The figure shows three views and two pictorial views of one solid part (mm, origin at its lowest corner). Answer the questions. Give positions to 0.01 mm unless a question says otherwise; leave off trailing zeros. Order: outer loops, then holes, each group sorted by start corner. A loop starts at its lowest first (then second) coordinate and runs counter-clockwise, first axis right, second up. Notation, with made-up numbers: (-19, -35) - (5, -35) arc R29 cw to (5, -15) - close; hole circle Ø5 at (1, 28). An arc over 180 degrees is marked (long way). Return JSON: item names as keys, results as strings. Group by question number.
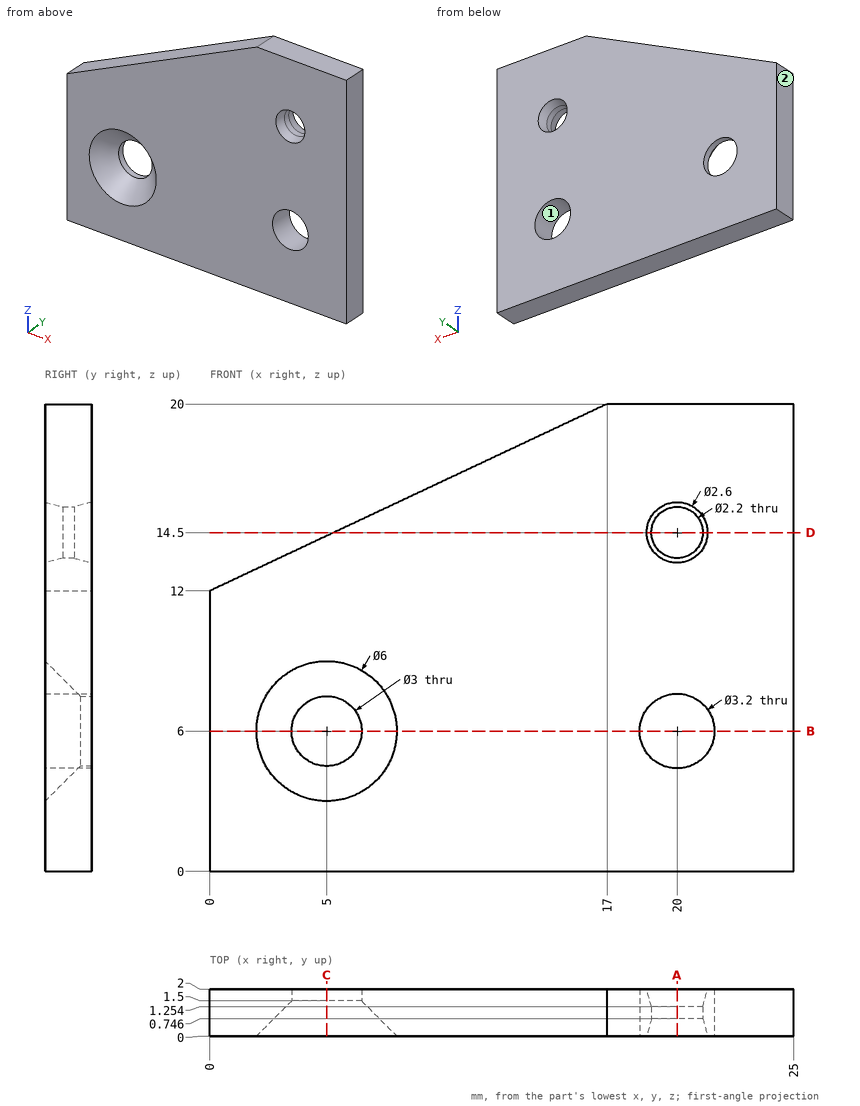
1. This flat-tipped pin is pushed along its axis until it touches: pin 1 (3 mm diameter, centred on x = 20, z = 14.5, fed in from +Y). Where does it stop, or does it pass through?
2. The part is cut by section D-D (z = 14.5). Give the vertices of the cut face in (x, y).
3. The part is cut by section A-A (x = 20). Give the vertices of the cut face in (y, z), and give its area (3 significant figures).
4. The part is cut by section C-C (x = 5). Give the vertices of the cut face in (y, z).
5. Determine the mould class of the marked faces 1 and 2 for opening direction Z: released by +Z, released by -Z, zero draft, split by the parting line, or undercut.
6. The part is cut by section B-B (z = 6). Give the vertices of the cut face in (x, y).
7. Consider probe 1 along X at (y, z) = (1.8, 6); probe 2 along X at (y, z) = (0.25, 5.25) (1 decimal); probe 3 along X at (y, z) = (1.1, 14.5) (1 decimal). Determine where each line is inside the solid, lowest interval first. Write a range as from..to.
Answers:
{
 "1": {"pin 1": "stops at y = 2"},
 "2": {"outline": "(5.31, 0) - (18.7, 0) - (18.9, 0.75) - (18.9, 1.25) - (18.7, 2) - (5.31, 2) - close; (21.1, 0.75) - (21.3, 0) - (25, 0) - (25, 2) - (21.3, 2) - (21.1, 1.25) - close"},
 "3": {"outline": "(0, 0) - (2, 0) - (2, 4.4) - (0, 4.4) - close; (0, 7.6) - (2, 7.6) - (2, 13.2) - (1.25, 13.4) - (0.75, 13.4) - (0, 13.2) - close; (0, 15.8) - (0.75, 15.6) - (1.25, 15.6) - (2, 15.8) - (2, 20) - (0, 20) - close", "area": "28.9 mm^2"},
 "4": {"outline": "(0, 0) - (2, 0) - (2, 4.5) - (1.5, 4.5) - (0, 3) - close; (0, 9) - (1.5, 7.5) - (2, 7.5) - (2, 14.35) - (0, 14.35) - close"},
 "5": {"face 1": "undercut", "face 2": "zero draft"},
 "6": {"outline": "(0, 0) - (2, 0) - (3.5, 1.5) - (3.5, 2) - (0, 2) - close; (6.5, 1.5) - (8, 0) - (18.4, 0) - (18.4, 2) - (6.5, 2) - close; (21.6, 0) - (25, 0) - (25, 2) - (21.6, 2) - close"},
 "7": {"probe 1": "x = 0..3.5, 6.5..18.4, 21.6..25", "probe 2": "x = 0..2.4, 7.6..18.6, 21.4..25", "probe 3": "x = 5.3..18.9, 21.1..25"}
}
